Can you work these out from the model? Positions are in its coordinate system, mm. Coordinates: 2 decimals unless noted, no trailing zeros. Order: outer loops, then holes, each group sorted by start corner. A loop starts at its lowest first (then second) coordinate and runs counter-clockwise, first axis right, second up. Notation, with made-up numbers: (51.25, 3) - (108.25, 3) arc R15 cw to (108.25, 10) - close; hole circle Ø5 at (30.25, 29). An arc over 180 degrees is marked (long way). Use a Markdown table: item, result. Add a question column.
(1) If I drill on L1, parallel to Z at x = -3, y = 0.8; L2, parallel to X at y = -0.8, z = 2; L3, parallel to Z at x = 7, y = -0.75, over which ranges is the centre line in solid material (lowest first)? Write a range as [from, to].
(2) I want a section at D-D (x = -15). List the corners of the cut face in (y, z) for me, and give its area (3 significant figures).
(3) For pin 1 Ø1.5 at (x, y) = (10.5, -1) entering from -Z; pin 2 Ø1.5 at (x, y) = (-4.5, 0) entering from -Z; pin 3 Ø2 at (x, y) = (-16.5, 0.5) entering from +Z, each with a flat end and sliding along its axis, tell me the tip position at first contact or that it passes through.
(4) I want a section at A-A (y = 1.45). List the corners of the cut face in (x, z) for me.
(5) I want a section at C-C (z = -6.25). List the corners of the cut face in (x, y) for me, and give its area (3 significant figures).
(6) I want a section at B-B (x = 9). List the corners of the cut face in (y, z) for me.
(7) We'd pull the mould along Z, two halves only. Please class faces 1 (the flat face through (-17, 0, 4.5)), 2 (the flat face through (-17, 0, -4.5)), 3 (the cylindrical face through (0.676, -0.028, 8.161)), 4 (the cylindrical face through (-11.02, -0.03, -6.8)): pulls with the +Z half, pulls with the -Z half, needs draft (parallel to the pull), parting line crosses it, or undercut.
```python
from build123d import *

# Parameters (mm, degrees)
SKETCH1_R           = 14.419595949
SKETCH1_R_2         = 5.55
SKETCH1_R_3         = 0.8
PLACA_CABEZAL_DEPTH = 4
SKETCH2_W           = 7.5
SKETCH2_H           = 9
PATA_AL_HUESO_DEPTH = 4


with BuildPart() as part:
    # Sketch1 → Placa_cabezal (new body)
    with BuildSketch(Plane(origin=(0, -2, 0), x_dir=(1, 0, 0), z_dir=(0, 1, 0))):
        with Locations(Location((0, 0, 0), (0, 0, 270))):
            Circle(SKETCH1_R)
        with Locations(Location((5.6, 5.6, 0), (0, 0, 270))):
            Circle(SKETCH1_R_2, mode=Mode.SUBTRACT)
        with Locations(Location((-5.6, 5.6, 0), (0, 0, 270))):
            Circle(SKETCH1_R_2, mode=Mode.SUBTRACT)
        with Locations(Location((-5.6, -5.6, 0), (0, 0, 270))):
            Circle(SKETCH1_R_2, mode=Mode.SUBTRACT)
        with Locations(Location((5.6, -5.6, 0), (0, 0, 270))):
            Circle(SKETCH1_R_2, mode=Mode.SUBTRACT)
        with Locations(Location((0, 0, 0), (0, 0, 270))):
            Circle(SKETCH1_R_3, mode=Mode.SUBTRACT)
    extrude(amount=PLACA_CABEZAL_DEPTH)

    # Sketch2 → Pata_al_hueso (add)
    with BuildSketch(Plane(origin=(0, -2, 0), x_dir=(1, 0, 0), z_dir=(0, 1, 0))):
        with Locations((-16.669595949, 0)):
            Rectangle(SKETCH2_W, SKETCH2_H)
    extrude(amount=PATA_AL_HUESO_DEPTH)


solid = part.part
```
Answers follow:
| question | item | result |
|---|---|---|
| 1 | L1 | z = [-14.1, -10.5], [-0.7, 0.7], [10.5, 14.1] |
| 1 | L2 | x = [-20.42, -9.82], [-1.38, 1.38], [9.82, 14.28] |
| 1 | L3 | z = [-12.61, -10.97], [-0.23, 0.23], [10.97, 12.61] |
| 2 | outline | (-2, -4.5) - (2, -4.5) - (2, 4.5) - (-2, 4.5) - close |
| 2 | area | 36.0 mm² |
| 3 | pin 1 | stops at z = -10.62 |
| 3 | pin 2 | stops at z = -13.92 |
| 3 | pin 3 | stops at z = 4.5 |
| 4 | outline | (-20.42, -4.5) - (-13.7, -4.5) arc R14.42 ccw (long way) to (-13.7, 4.5) - (-20.42, 4.5) - close; hole circle Ø11.1 at (-5.6, -5.6); hole circle Ø11.1 at (-5.6, 5.6); hole circle Ø1.6 at (0, 0); hole circle Ø11.1 at (5.6, -5.6); hole circle Ø11.1 at (5.6, 5.6) |
| 5 | outline | (-12.99, -2) - (-11.11, -2) - (-11.11, 2) - (-12.99, 2) - close; (-0.09, -2) - (0.09, -2) - (0.09, 2) - (-0.09, 2) - close; (11.11, -2) - (12.99, -2) - (12.99, 2) - (11.11, 2) - close |
| 5 | area | 15.8 mm² |
| 6 | outline | (-2, -11.27) - (2, -11.27) - (2, -9.99) - (-2, -9.99) - close; (-2, -1.21) - (2, -1.21) - (2, 1.21) - (-2, 1.21) - close; (-2, 9.99) - (2, 9.99) - (2, 11.27) - (-2, 11.27) - close |
| 7 | face 1 | pulls with the +Z half |
| 7 | face 2 | pulls with the -Z half |
| 7 | face 3 | undercut |
| 7 | face 4 | undercut |
